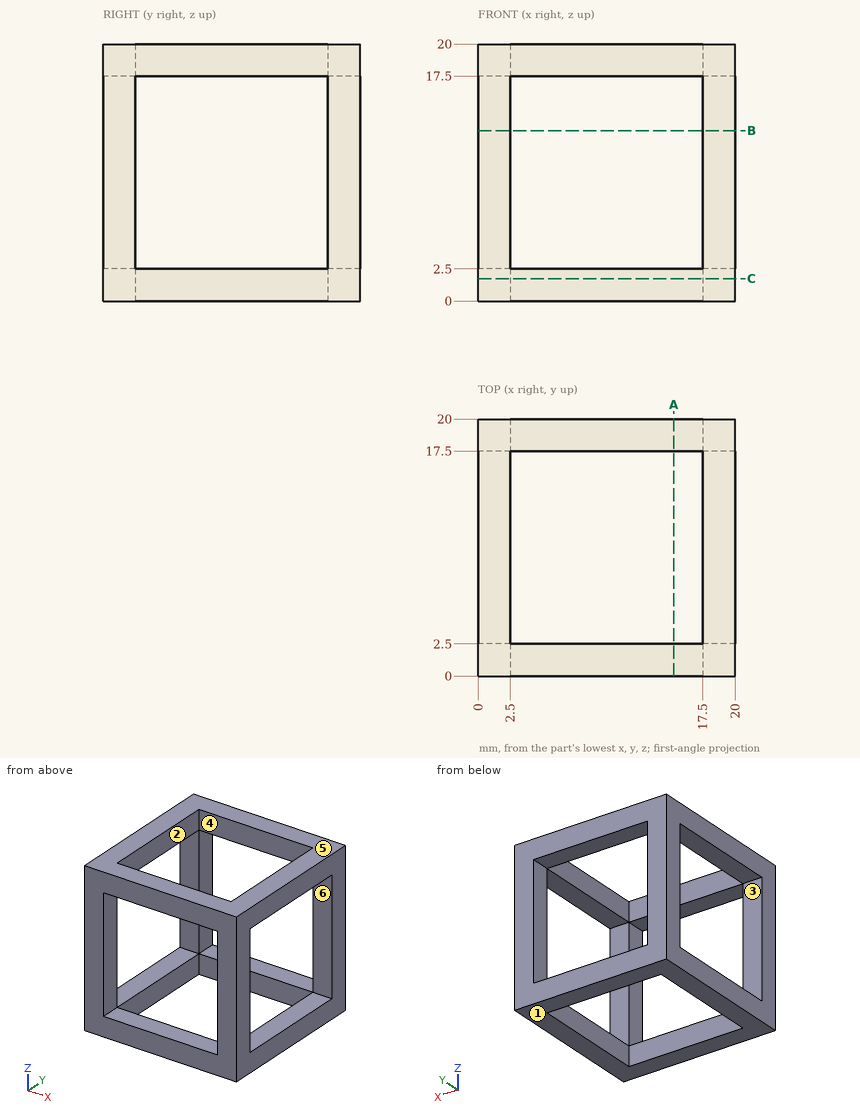
Drawing for the job (mm, zero at the part's lowest x, y, z). A direction names the side the tool comes from. Round coordinates to 2 decimals unless told otherwise and drop trailing zeros. Loops run counter-clockwise (first coordinate to the right, second up) from the corner with the lowest first, then second, coordinate; pieces in that order, holes last. Notation, with made-up numbers: M -17,-4.75 L 20,-4.75 A20 ccw 20,20.25 Z; hole C 17.25,44 d8. An arc over 180 degrees is marked long. Use a Markdown table: item, result. Add a question column.
(1) Cut at C-C (z = 1.75). Give the cut face in (x, y), and give its area (3 significant figures).
(2) Flat gauge pins, fed straight in: pin 1 (1 mm diameter, centred on x = 6.5, y = 2.5, fed in from -Z); pin 2 (8 mm diameter, centred on x = 11.5, y = 7.5, fed in from +Z). Where does each tip first touch, or does it go through?
(3) Cut at A-A (x = 15.25). Give the cut face in (y, z).
(4) Pull direction Z, two halves, no side cores. Call the marked faces 1, 2 and 3: +Z half, -Z half, draft (parallel to the pull), parting line (faces both ways), or undercut.
(5) Which spindle directions (+Z, -Z, +X, -X, +Y, -Y) get a long thin tool onto all of the face, cutting with end or side? Do the marked faces 4, 5 and 6. Say none if no direction does.
(6) Drill centre line: line 1 (X direction, y = 4.5, z = 1). Where is it in solid material? Low to high.
Geometry says:
| question | item | result |
|---|---|---|
| 1 | outline | M 0,0 L 20,0 L 20,20 L 0,20 Z; hole M 2.5,2.5 L 17.5,2.5 L 17.5,17.5 L 2.5,17.5 Z |
| 1 | area | 175 mm² |
| 2 | pin 1 | stops at z = 0 |
| 2 | pin 2 | passes through |
| 3 | outline | M 0,0 L 2.5,0 L 2.5,2.5 L 0,2.5 Z; M 0,17.5 L 2.5,17.5 L 2.5,20 L 0,20 Z; M 17.5,0 L 20,0 L 20,2.5 L 17.5,2.5 Z; M 17.5,17.5 L 20,17.5 L 20,20 L 17.5,20 Z |
| 4 | face 1 | -Z half |
| 4 | face 2 | draft |
| 4 | face 3 | undercut |
| 5 | face 4 | +Z, -Z |
| 5 | face 5 | +Z, +X, -X, +Y, -Y |
| 5 | face 6 | +X, -X |
| 6 | line 1 | x = 0 to 2.5, 17.5 to 20 |
